Source: CAD feature listing. Evaluate the final solid. Frame: model axes, mm. A direction names the side the tool comes from. Round coordinates to 2 decimals unless told otherwise and drop trailing zeros. Loops run counter-clockwise (first coordinate to the right, second up) from the corner with the lowest first, then second, coordinate; pieces in that order, holes last.
Item 1: First-contact query: P1, Ø5, axis at x = 87, z = 46.5, coming from the +Y side; P2, Ø2, axis at y = 2.5, z = 55.5, coming from the -X side; P3, Ø8, axis at x = 50, z = 53, coming from the +Y side; P4, Ø2, axis at x = 101, y = 0.5, coming from the -Z side. Flat tips, straight axial feed; report the tip coordinate or a pass-through.
Item 2: Section query B-B on z = 48. Return loops of the section in (x, y).
Item 3: Ray query, L1, parallel to Z at x = 50, y = 1.7; L2, parallel to X at y = 1.15, z = 21; L3, parallel to Z at x = 109, y = 2.6. Return the intervals inside material, ascending.
Item 4: Section query A-A on x = 91.5. Return loops of the section in (y, z).
Item 5: Section query D-D on x = 68. Return loops of the section in (y, z).
Item 6: Section query C-C on y = 2.2. Give the number of separate pieces and of enclosed holes in the cut face, then the cut area to 3 significant figures.
Item 7: Pull-direction query (Z, two-part tool) for faces 1 (the flat face through (49.5, 2, 2)), 2 (the flat face through (44, 2, 4)), 3 (the flat face through (83, 2, 23.5)), 4 (the flat face through (2, 2, 32)); classes: released by +Z, released by -Z, zero draft, split by the parting line, or undercut.
Item 8: Access query for faces 5 (the flat face through (109, 2, 54)), 6 (the flat face through (79.5, 2, 2)), 7 (the flat face through (125, 2, 17)), 8 (the flat face through (2, 2, 12)). Directions: +Z, -Z, +X, -X, +Y, -Y. A direction counts if a zero-diameter tool reaches every point of the face in a straight line with its end or side. Return the directions, or none.
```python
from build123d import *

# Parameters (mm, degrees)
SKETCH1_W           = 129
SKETCH1_H           = 74
BOSS_EXTRUDE1_DEPTH = 4
SKETCH2_R           = 3.5
SKETCH2_W           = 19
SKETCH2_H           = 27
CUT_EXTRUDE1_DEPTH  = 5
SKETCH3_W           = 5
SKETCH3_H           = 2
CUT_EXTRUDE2_DEPTH  = 5
SKETCH4_W           = 4
SKETCH4_H           = 10
SKETCH4_W_2         = 10
SKETCH4_H_2         = 4
CUT_EXTRUDE3_DEPTH  = 5


with BuildPart() as part:
    # Sketch1 → Boss-Extrude1 (new body)
    with BuildSketch(Plane(origin=(0, 0, 0), x_dir=(1, 0, 0), z_dir=(0, 1, 0))):
        with Locations((64.5, -37)):
            Rectangle(SKETCH1_W, SKETCH1_H)
    extrude(amount=BOSS_EXTRUDE1_DEPTH)

    # Sketch2 → Cut-Extrude1 (cut, through all)
    with BuildSketch(Plane(origin=(0, 4, 0), x_dir=(1, 0, 0), z_dir=(0, 1, 0))):
        with Locations((50, -21)):
            Circle(SKETCH2_R)
        with Locations((50, -53)):
            Circle(SKETCH2_R)
        with Locations((83.5, -37)):
            Rectangle(SKETCH2_W, SKETCH2_H)
    extrude(amount=-CUT_EXTRUDE1_DEPTH, mode=Mode.SUBTRACT)

    # Sketch3 → Cut-Extrude2 (cut, through all)
    with BuildSketch(Plane(origin=(0, 4, 0), x_dir=(1, 0, 0), z_dir=(0, 1, 0))):
        with Locations((109, -21)):
            Rectangle(SKETCH3_W, SKETCH3_H)
        with Locations((109, -53)):
            Rectangle(SKETCH3_W, SKETCH3_H)
    extrude(amount=-CUT_EXTRUDE2_DEPTH, mode=Mode.SUBTRACT)

    # Sketch4 → Cut-Extrude3 (cut, through all)
    with BuildSketch(Plane(origin=(0, 4, 0), x_dir=(1, 0, 0), z_dir=(0, 1, 0))):
        with Locations((127, -57)):
            Rectangle(SKETCH4_W, SKETCH4_H)
        with Locations((127, -37)):
            Rectangle(SKETCH4_W, SKETCH4_H)
        with Locations((127, -17)):
            Rectangle(SKETCH4_W, SKETCH4_H)
        with Locations((2, -57)):
            Rectangle(SKETCH4_W, SKETCH4_H)
        with Locations((2, -37)):
            Rectangle(SKETCH4_W, SKETCH4_H)
        with Locations((2, -17)):
            Rectangle(SKETCH4_W, SKETCH4_H)
        with Locations((104.5, -2)):
            Rectangle(SKETCH4_W_2, SKETCH4_H_2)
        with Locations((84.5, -2)):
            Rectangle(SKETCH4_W_2, SKETCH4_H_2)
        with Locations((64.5, -2)):
            Rectangle(SKETCH4_W_2, SKETCH4_H_2)
        with Locations((44.5, -2)):
            Rectangle(SKETCH4_W_2, SKETCH4_H_2)
        with Locations((24.5, -2)):
            Rectangle(SKETCH4_W_2, SKETCH4_H_2)
        with Locations((104.5, -72)):
            Rectangle(SKETCH4_W_2, SKETCH4_H_2)
        with Locations((84.5, -72)):
            Rectangle(SKETCH4_W_2, SKETCH4_H_2)
        with Locations((64.5, -72)):
            Rectangle(SKETCH4_W_2, SKETCH4_H_2)
        with Locations((44.5, -72)):
            Rectangle(SKETCH4_W_2, SKETCH4_H_2)
        with Locations((24.5, -72)):
            Rectangle(SKETCH4_W_2, SKETCH4_H_2)
    extrude(amount=-CUT_EXTRUDE3_DEPTH, mode=Mode.SUBTRACT)


solid = part.part
```
Data:
1. P1: passes through
1. P2: stops at x = 4
1. P3: stops at y = 4
1. P4: stops at z = 4
2. outline: (0, 0) - (74, 0) - (74, 4) - (0, 4) - close; (93, 0) - (129, 0) - (129, 4) - (93, 4) - close
3. L1: z = 0 to 17.5, 24.5 to 49.5, 56.5 to 74
3. L2: x = 4 to 46.5, 53.5 to 106.5, 111.5 to 125
3. L3: z = 4 to 20, 22 to 52, 54 to 70
4. outline: (0, 0) - (4, 0) - (4, 23.5) - (0, 23.5) - close; (0, 50.5) - (4, 50.5) - (4, 74) - (0, 74) - close
5. outline: (0, 4) - (4, 4) - (4, 70) - (0, 70) - close
6. separate pieces: 1
6. enclosed holes: 5
6. area: 8,300 mm2
7. face 1: zero draft
7. face 2: released by -Z
7. face 3: undercut
7. face 4: undercut
8. face 5: +Y, -Y
8. face 6: -Z, +Y, -Y
8. face 7: +X, +Y, -Y
8. face 8: -X, +Y, -Y
